Answer from the drawing. Dimensions are ordinates in mm from the lowest x, y and z of the part. A direction names the side the tool comes from. Coordinates: 2 decimals unless noted, no trailing zeros. Write each loop counter-clockwise with the first axis right and the second up, starting at its lowest first coordinate (ties: lowest second). Pieces come first, ordered by that corner, then holes.
(1) The part is cut by section D-D, the plane y = 27.5. Determine the outline of the cut face in (x, z), and give its area (3 significant figures).
(2) Given pin 1 (6 mm diameter, centred on x = 37.5, z = 33.5, fed in from +Y); pin 2 (4.5 mm diameter, centred on x = 4, y = 4, fed in from +Z); pin 3 (3 mm diameter, centred on x = 15, y = 44.5, fed in from -Z), each flat-ended and moving along its own axis, determine where each tip first touches the part or whether it passes through.
(3) Which of the six approach directions +Z, -Z, +X, -X, +Y, -Y give full straight-line access (tool end or side, diameter ignored) to the marked faces 1 and 2?
(4) The part is cut by section A-A, the plane y = 4. Determine the outline of the cut face in (x, z), and give its area (3 significant figures).
(5) The part is cut by section C-C, the plane x = 30. Determine the outline of the cut face in (y, z), and give its area (3 significant figures).
(6) Straight lines are drawn through the part: line 1 along Y through (x, z) = (4, 15); line 2 along Z through (x, y) = (55, 52); line 3 along Y through (x, z) = (26.5, 33). For each, find the intervals that lie inside material, in ascending order.
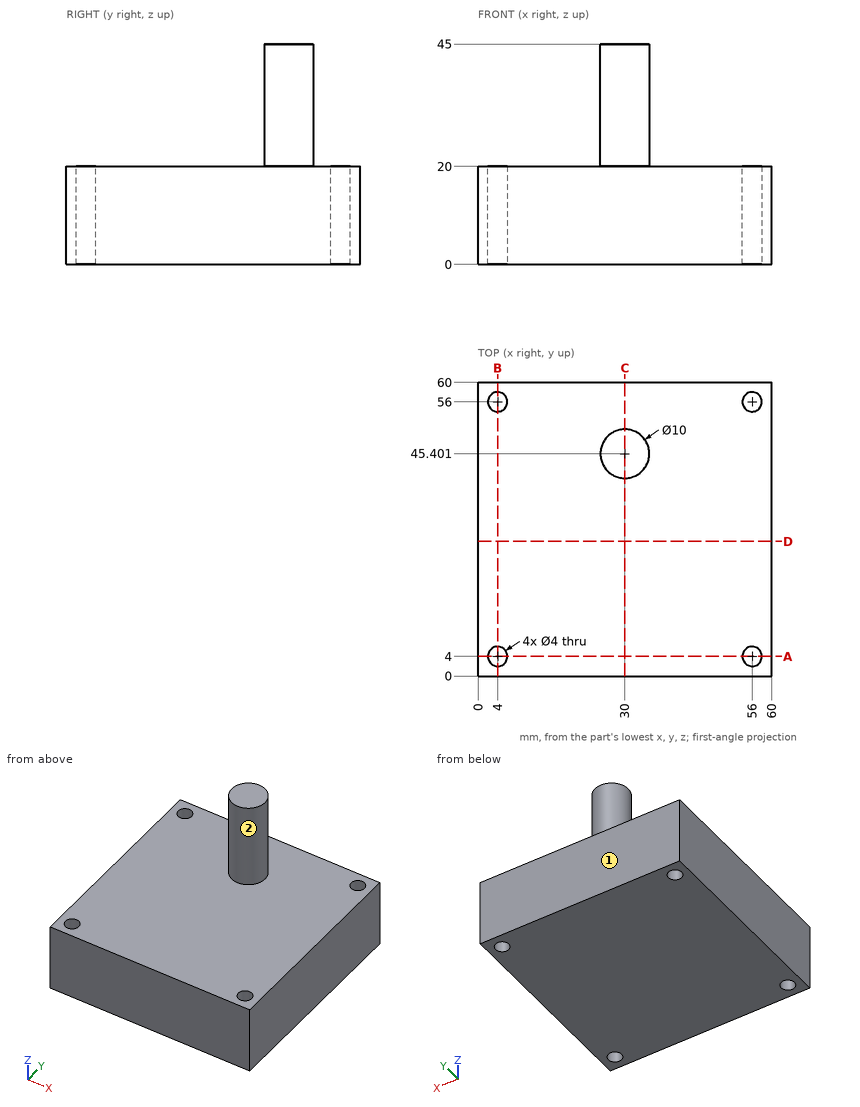
Computed:
1. outline: (0, 0) - (60, 0) - (60, 20) - (0, 20) - close
1. area: 1,200 mm2
2. pin 1: stops at y = 47.58
2. pin 2: stops at z = 20
2. pin 3: stops at z = 0
3. face 1: +Z, -Z, +X, -X, +Y
3. face 2: +Z
4. outline: (0, 0) - (2, 0) - (2, 20) - (0, 20) - close; (6, 0) - (54, 0) - (54, 20) - (6, 20) - close; (58, 0) - (60, 0) - (60, 20) - (58, 20) - close
4. area: 1,040 mm2
5. outline: (0, 0) - (60, 0) - (60, 20) - (50.4, 20) - (50.4, 45) - (40.4, 45) - (40.4, 20) - (0, 20) - close
5. area: 1,450 mm2
6. line 1: y = 0 to 2, 6 to 54, 58 to 60
6. line 2: z = 0 to 20
6. line 3: y = 41.83 to 48.97
